from build123d import *

# Parameters (mm, degrees)
SKETCH1_R           = 11
BOSS_EXTRUDE1_DEPTH = 27.1
SKETCH2_R           = 12.5
BOSS_EXTRUDE2_DEPTH = 1.3
SKETCH3_R           = 6
CUT_EXTRUDE1_DEPTH  = 29.3


with BuildPart() as part:
    # Sketch1 → Boss-Extrude1 (new body)
    with BuildSketch(Plane(origin=(0, 0, 0), x_dir=(1, 0, 0), z_dir=(0, 1, 0))):
        with Locations(Location((0, 0, 0), (0, 0, 90))):
            Circle(SKETCH1_R)
    extrude(amount=BOSS_EXTRUDE1_DEPTH)

    # Sketch2 → Boss-Extrude2 (add)
    with BuildSketch(Plane(origin=(0, 0, 0), x_dir=(1, 0, 0), z_dir=(0, 1, 0))):
        with Locations(Location((0, 0, 0), (0, 0, 270))):
            Circle(SKETCH2_R)
    extrude(amount=BOSS_EXTRUDE2_DEPTH)

    # Sketch3 → Cut-Extrude1 (cut)
    with BuildSketch(Plane(origin=(0, 0, 0), x_dir=(1, 0, 0), z_dir=(0, 1, 0))):
        with Locations(Location((0, 0, 0), (0, 0, 270))):
            Circle(SKETCH3_R)
    extrude(amount=CUT_EXTRUDE1_DEPTH, mode=Mode.SUBTRACT)


solid = part.part
Build history of the part. All positions in model axes, mm. Round coordinates to 2 decimals unless told otherwise and drop trailing zeros. Write each loop counter-clockwise with the first axis right and the second up, starting at its lowest first coordinate (ties: lowest second). Pieces come first, ordered by that corner, then holes. Notation, with made-up numbers: M 48,75 L 92,75 A26 ccw 92,91 Z; hole C -7.5,61 d7. An arc over 180 degrees is marked long. Answer as a JSON object with one key per item and string values. Group by question number.
(1) Cut at B-B (z = 0). Give the cut face in (x, y).
(2) Flat gauge pins, fed straight in: pin 1 (10 mm diameter, centred on x = -9, y = 12, fed in from -Z); pin 2 (10 mm diameter, centred on x = 0.5, y = 15.5, fed in from +Z); pin 3 (12 mm diameter, centred on y = 9, z = 1.5, fed in from +X). Where does each tip first touch, or does it go through?
(3) Mould opens along X. For faces 1 (the flat face through (-10, 1.3, 5)), 2 (the cylindrical face through (10.74, 14.02, 2.38)), 3 (the cylindrical face through (1.802, 13.36, 5.723)) say: pulls with the +X half, pulls with the -X half, needs draft (parallel to the pull), parting line crosses it, or undercut.
(4) Cut at C-C (y = 23.5). Give the cut face in (x, z).
(5) Drill centre lines: L1, parallel to X at y = 6, z = 0; L2, parallel to X at y = 3, z = -2.25; L3, parallel to Z at x = 4, y = 10.5. Where is each one in solid material? Low to high.
(6) Cut at A-A (x = 0). Give the cut face in (y, z).
(7) Cut at D-D (z = -8.5). Give the cut face in (x, y).
Responses:
{
 "1": {"outline": "M -12.5,0 L -6,0 L -6,27.1 L -11,27.1 L -11,1.3 L -12.5,1.3 Z; M 6,0 L 12.5,0 L 12.5,1.3 L 11,1.3 L 11,27.1 L 6,27.1 Z"},
 "2": {"pin 1": "stops at z = -10.25", "pin 2": "stops at z = 11", "pin 3": "stops at x = 11"},
 "3": {"face 1": "needs draft", "face 2": "parting line crosses it", "face 3": "undercut"},
 "4": {"outline": "C 0,0 d22; hole C 0,0 d12"},
 "5": {"L1": "x = -11 to -6, 6 to 11", "L2": "x = -10.77 to -5.56, 5.56 to 10.77", "L3": "z = -10.25 to -4.47, 4.47 to 10.25"},
 "6": {"outline": "M 0,-12.5 L 1.3,-12.5 L 1.3,-11 L 27.1,-11 L 27.1,-6 L 0,-6 Z; M 0,6 L 27.1,6 L 27.1,11 L 1.3,11 L 1.3,12.5 L 0,12.5 Z"},
 "7": {"outline": "M -9.17,0 L 9.17,0 L 9.17,1.3 L 6.98,1.3 L 6.98,27.1 L -6.98,27.1 L -6.98,1.3 L -9.17,1.3 Z"}
}
